Geometry check sheet. Reference: the model listing, model coordinates, mm. Face numbers are marked on the shaded views. Coordinates: 2 decimals unless noted, no trailing zeros. Order: outer loops, then holes, each group sorted by start corner. A loop starts at its lowest first (then second) coordinate and runs counter-clockwise, first axis right, second up. Notation, with made-up numbers: (60, 61.25) - (113, 61.25) arc R30 ccw to (113, 93.25) - close; hole circle Ø9 at (72.25, 15.5). An arc over 180 degrees is marked (long way). Put each result on its own line as item: value.
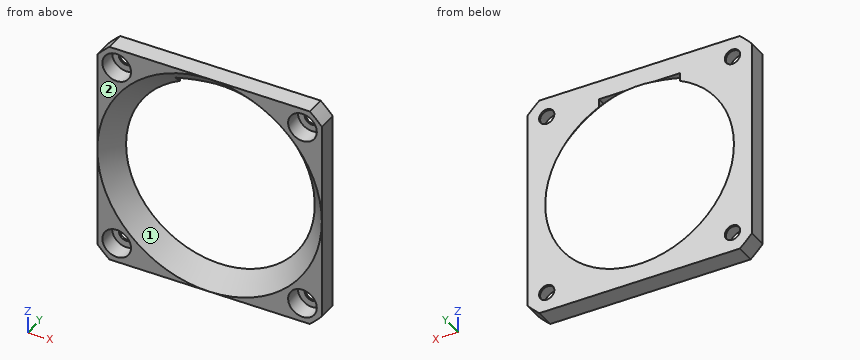
from build123d import *

# Parameters (mm, degrees)
SKETCH1_R         = 31.5
SKETCH1_R_2       = 1.6
BASE_DEPTH        = 4
SKETCH3_R         = 23.5
SKETCH4_R         = 19.75054858
CONNECTORS_DEPTH  = 45.72694938
SKETCH5_R         = 3
SCREW_HEADS_DEPTH = 3.6
FLEX_CABLE_DEPTH  = 34.473870559


with BuildPart() as part:
    # Sketch1 → Base (new body)
    with BuildSketch(Plane(origin=(0, 0, 0), x_dir=(1, 0, 0), z_dir=(0, 1, 0))):
        with Locations(Location((0, 0, 0), (0, 0, 270))):
            Circle(SKETCH1_R)
        with Locations(Location((-19.445436483, -19.445436483, 0), (0, 0, 270))):
            Circle(SKETCH1_R_2, mode=Mode.SUBTRACT)
        with Locations(Location((-19.445436483, 19.445436483, 0), (0, 0, 270))):
            Circle(SKETCH1_R_2, mode=Mode.SUBTRACT)
        with Locations(Location((19.445436483, -19.445436483, 0), (0, 0, 270))):
            Circle(SKETCH1_R_2, mode=Mode.SUBTRACT)
        with Locations(Location((19.445436483, 19.445436483, 0), (0, 0, 270))):
            Circle(SKETCH1_R_2, mode=Mode.SUBTRACT)
    extrude(amount=-BASE_DEPTH)

    # Sketch3 → Skirt section 0
    with BuildSketch(Plane(origin=(0, -4, 0), x_dir=(-1, 0, 0), z_dir=(0, -1, 0))):
        Circle(SKETCH3_R)
    # Sketch4 → Skirt section 1
    with BuildSketch(Plane(origin=(0, 0, 0), x_dir=(1, 0, 0), z_dir=(0, 1, 0))):
        Circle(SKETCH4_R)
    loft(mode=Mode.SUBTRACT)

    # Sketch6 → Connectors (cut, through all)
    with BuildSketch(Plane(origin=(0, -4, 0), x_dir=(-1, 0, 0), z_dir=(0, -1, 0))):
        with BuildLine():
            Line((20.976176963, 23.5), (-20.976176963, 23.5))
            ThreePointArc((-20.976176963, 23.5), (0, 31.5), (20.976176963, 23.5))
        make_face()
        with BuildLine():
            Line((20.976176963, -23.5), (-20.976176963, -23.5))
            ThreePointArc((-20.976176963, -23.5), (0, -31.5), (20.976176963, -23.5))
        make_face()
        with BuildLine():
            Line((23.5, -20.976176963), (23.5, 20.976176963))
            ThreePointArc((23.5, 20.976176963), (31.5, 0), (23.5, -20.976176963))
        make_face()
        with BuildLine():
            Line((-23.5, -20.976176963), (-23.5, 20.976176963))
            ThreePointArc((-23.5, 20.976176963), (-31.5, 0), (-23.5, -20.976176963))
        make_face()
    extrude(amount=-CONNECTORS_DEPTH, mode=Mode.SUBTRACT)

    # Sketch5 → Screw heads (cut)
    with BuildSketch(Plane(origin=(0, -4, 0), x_dir=(-1, 0, 0), z_dir=(0, -1, 0))):
        with Locations(Location((19.445436483, -19.445436483, 0), (0, 0, 90))):
            Circle(SKETCH5_R)
        with Locations(Location((19.445436483, 19.445436483, 0), (0, 0, 90))):
            Circle(SKETCH5_R)
        with Locations(Location((-19.445436483, -19.445436483, 0), (0, 0, 90))):
            Circle(SKETCH5_R)
        with Locations(Location((-19.445436483, 19.445436483, 0), (0, 0, 90))):
            Circle(SKETCH5_R)
    extrude(amount=-SCREW_HEADS_DEPTH, mode=Mode.SUBTRACT)

    # Sketch7 → Flex cable (cut, through all)
    with BuildSketch(Plane(origin=(0, 0, 0), x_dir=(1, 0, 0), z_dir=(0, 1, 0))):
        Polygon((-8.5, -19.55054858), (8.5, -19.55054858), (8.5, -18.75054858), (8.5, 0), (0, 0), (-8.5, 0), (-8.5, -18.75054858), align=None)
    extrude(amount=-FLEX_CABLE_DEPTH, mode=Mode.SUBTRACT)


solid = part.part
Q1. Draft check along X on the marked faces 1 and 2. Enter one of: pulls with the +X half, pulls with the -X half, needs draft (parallel to the pull), parting line crosses it, or undercut.
Answer block:
face 1: undercut
face 2: needs draft
Q2. Section check B-B on z = -19.5. State how many separate pieces and enclosed holes the cut face has, then the cut area to 3 significant figures.
Answer block:
separate pieces: 4
enclosed holes: 0
area: 70.2 mm^2
Q3. Thickness scan on L1, parallel to Z at x = 17, y = -2.4; L2, parallel to X at y = -3, z = -19; L3, parallel to Z at x = 15.5, y = -3.05. Record the ranges inside material, lowest first. Write a range as [from, to].
Answer block:
L1: z = [-23.5, -21.18], [-17.71, -13.96], [13.96, 17.71], [21.18, 23.5]
L2: x = [-23.5, -22.41], [-16.48, -12.17], [12.17, 16.48], [22.41, 23.5]
L3: z = [-23.5, -16.46], [16.46, 23.5]
Q4. Depth check by flat-ended pin: pin 1 Ø3 at (x, z) = (18.5, -19) entering from -Y; pin 2 Ø1.9 at (x, z) = (-19.45, -19.45) entering from -Y. Enter the tip coordinate at first touch or a pass-through.
Answer block:
pin 1: stops at y = -0.4
pin 2: passes through
Q5. Section check A-A on y = -3.15. Record the boundary of the cut face in (x, z).
Answer block:
outline: (-23.5, -20.98) arc R31.5 ccw to (-20.98, -23.5) - (20.98, -23.5) arc R31.5 ccw to (23.5, -20.98) - (23.5, 20.98) arc R31.5 ccw to (20.98, 23.5) - (-20.98, 23.5) arc R31.5 ccw to (-23.5, 20.98) - close; hole circle Ø45.41 at (0, 0); hole circle Ø6 at (-19.45, -19.45); hole circle Ø6 at (-19.45, 19.45); hole circle Ø6 at (19.45, -19.45); hole circle Ø6 at (19.45, 19.45)
